Input: part model. Units: mm. Frame: model coordinates. A direction names the side the tool comes from. Round coordinates to 2 decimals unless told otherwise and drop trailing zeros. Loops run counter-clockwise (first coordinate to the right, second up) from the corner with the lowest first, then second, coordinate; pieces in that order, holes last. Notation, with made-up numbers: M -13.75,-24.5 L 44.25,-24.5 A26 ccw 44.25,5.5 Z; hole C 42,25 d4. An arc over 180 degrees is marked long. Use one line per item in the form item = value. Start each with the question number.
Q1. First-contact query: P1, Ø2.5, axis at y = 0, z = 0, coming from the -X side; P2, Ø2, axis at x = 5.5, z = 0.5, coming from the +Y side. Flat tips, straight axial feed; report the tip coordinate or a pass-through.
Q2. Mould query, pull axis Y, two halves, no side actions, for faces 1 (the conical face through (0.076, -3.632, 0.009)), 2 (the conical face through (3.833, -0.275, -0.061)), 3 (the conical face through (0.076, 3.632, -0.009)). Classes: pulls with the +Y half, pulls with the -Y half, needs draft (parallel to the pull), parting line crosses it, or undercut.
Q3. Ray query, line 1 along Z through (x, y) = (1.8, 0); line 2 along X through (y, z) = (0.5, 3.25); line 3 along Y through (x, z) = (3, 1.25). Return the intervals inside material, ascending.
Q4. Section query B-B, the plane x = 5.5. Output: boundary loops of the cut face in (y, z) (1 decimal), and give its area (3 significant figures).
Q5. Access query for faces 4 (the cylindrical face through (1.659, 1.438, 0.748)), 5 (the flat face through (2, 0, -3.5)), 6 (the cylindrical face through (3.989, -2.539, 1.947)). Directions: +Z, -Z, +X, -X, +Y, -Y. A direction counts if a zero-diameter tool reaches every point of the face in a straight line with its end or side. Return the directions, or none.
Q6. Section query A-A, the plane x = 1.75. Output: boundary loops of the cut face in (y, z).
Autodesk Inventor part; units mm, degrees
ref_plane "Work Plane1" through (1.53, 0, 0) normal (0, 0.866, -0.5) x (-1, 0, 0)
ref_plane "YZ Plane" through (0, 0, 0) normal (1, 0, 0) x (0, 1, 0)
ref_plane "XZ Plane" through (0, 0, 0) normal (0, 1, 0) x (-1, 0, 0)
sketch "Эскиз1" plane through (0, 0, 0) normal (1, 0, 0) x (0, 1, 0)
  line L0 (-2.0207, -3.5) -> (-4.0415, 0)
  line L1 (-4.0415, 0) -> (-2.0207, 3.5)
  line L2 (-2.0207, 3.5) -> (2.0207, 3.5)
  line L3 (2.0207, 3.5) -> (4.0415, 0)
  line L4 (4.0415, 0) -> (2.0207, -3.5)
  line L5 (2.0207, -3.5) -> (-2.0207, -3.5)
  point P0 (0, 0)
  point P1 (0, 0)
  dimension "d0" = 8.0829
extrude "Базовый элемент" add sketch "Эскиз1" along normal blind 3.2
sketch "Эскиз2" plane through (0, 0, 0) normal (0, 0, 1) x (1, 0, 0)
  line L0 (3.2, 0) -> (8, 0)
  arc A0 (8, 0) -> (4.8, 3.2) centre (4.8, 0) ccw
  line L1 (4.8, 3.2) -> (3.2, 3.2)
  line L2 (3.2, -2.0207) -> (3.2, 2.0207)
  line L3 (3.2, 0) -> (3.2, 3.2)
  line L4 (2.1075, 0) -> (9.7553, 0)
  dimension "d8" = 3.2
  dimension "d9" = 4.8
revolve "Наконечник" add sketch "Эскиз2" angle 360 about axis through (3.2, 0, 0) along (1, 0, 0)
sketch "Эскиз3" plane through (0, 0, 0) normal (-1, 0, 0) x (0, 0, 1)
  line L0 (0, -5.658) -> (0, 5.658)
  line L1 (-4.9, 0) -> (4.9, 0)
  point P0 (0, 0)
hole "Резьба" at (0, 0, 0) direction (1, 0, 0) diameter 3.242 depth 3.06 tip angle 120
sketch "Эскиз4" plane through (0, 0, 0) normal (0, 0, 1) x (1, 0, 0)
  line L0 (0, 2.0207) -> (0, 4.0415)
  line L1 (0, 4.0415) -> (3.2, 4.0415)
  line L2 (3.2, 2.0207) -> (3.2, 4.0415)
  line L3 (-0.64, 0) -> (3.84, 0)
  line L4 (0.3126, 4.0415) -> (0, 3.5)
  line L5 (2.8874, 4.0415) -> (3.2, 3.5)
  dimension "d3" = 7
  dimension "d4" = 30
  dimension "d5" = 7
  dimension "d6" = 30
revolve "Фаска1" cut sketch "Эскиз4" angle 360 about axis through (-10, 0, 0) along (1, 0, 0)
chamfer "Фаска2" distance 0.3789 angle 30 1 edges at (0, 0, -1.621) measured on face at (0, -2.8569, 0.0651)
ref_plane "Work Plane1" through (1.53, 0, 0) normal (0, 0.866, -0.5) x (-1, 0, 0)
equation "\"d0\" = 1.1547 * SW"
equation "\"d1\" = SIH"
equation "\"d8\" = KR"
equation "\"d9\" = KOH1 - SIH"
equation "\"d11\" = GEL"
equation "\"d12\" = 1.02 * GEL"
equation "\"d3\" = SW0"
equation "\"d4\" = ANG1"
equation "\"d5\" = SW01"
equation "\"d6\" = ANG2"
equation "\"d14\" = -0.5 * GD1 + 0.5 * NND"
equation "\"d36\" = -0.5 * GD1 + 0.5 * NND"
equation "\"ANG1\" = 30deg"
equation "\"ANG2\" = 30deg"
equation "\"NND\" = 4"
equation "\"SIH\" = 3.2"
equation "\"KOH1\" = 8"
equation "\"GEL\" = 3"
equation "\"SW\" = 7"
equation "\"KR\" = 3.2"
equation "\"SW0\" = SW"
equation "\"SW01\" = SW"
equation "\"GUL\" = 0.541266 * PTC"
equation "\"THREADDIA\" = 4"
equation "\"SDH\" = 6"
equation "\"TOA\" = 30deg"
equation "\"PTC\" = 0.7"
equation "\"E0\" = 1.155 * SW"
equation "\"GAL\" = 0.541266 * PTC"
properties part number "Гайка M4-6H ГОСТ 11860-85" material "Сталь, мягкая"
Results found:
q1.P1 = 3.27
q1.P2 = 3.2
q2.face_1 = pulls with the -Y half
q2.face_2 = undercut
q2.face_3 = pulls with the +Y half
q3.line_1 = -3.5 to -1.62, 1.62 to 3.5
q3.line_2 = 0 to 3.2
q3.line_3 = -3.32 to -1.03, 1.03 to 3.32
q4.outline = C 0,0 d6.2
q4.area = 30.6 mm²
q5.face_4 = -X
q5.face_5 = -Z, +X, -X, +Y, -Y
q5.face_6 = +X
q6.outline = M -4.04,0 L -2.02,-3.5 L 2.02,-3.5 L 4.04,0 L 2.02,3.5 L -2.02,3.5 Z; hole C 0,0 d3.24
